Can you work these out from the model? Positions are in its coordinate system, mm. Face numbers are marked on the shaded views. A direction names the side the tool comes from. Coordinates: 2 decimals unless noted, no trailing zeros. Loops run counter-clockwise (first coordinate to the right, second up) from the corner with the lowest first, then second, coordinate; pieces in that order, holes last.
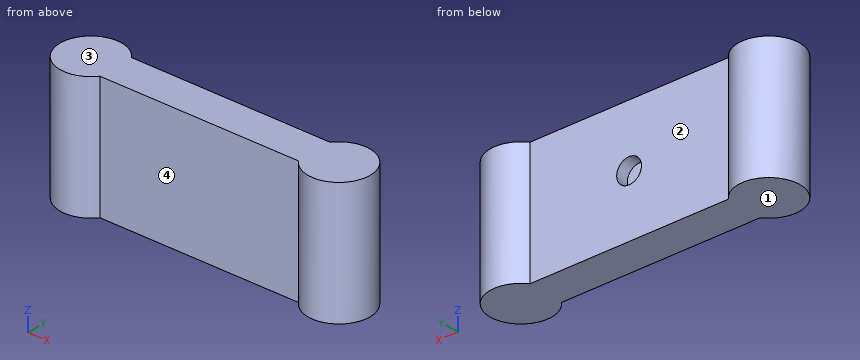
```python
from build123d import *

# Parameters (mm, degrees)
F0_W     = 200
F0_H     = 100
F1_DEPTH = 30
F2_R     = 25
F3_DEPTH = 50
F4_R     = 10
F5_DEPTH = 10


with BuildPart() as f1:
    # F0 (on Front) → F1 (new body)
    with BuildSketch(Plane.XZ):
        Rectangle(F0_W, F0_H)
    extrude(amount=F1_DEPTH)

    # F2 (on Top) → F3 (join, symmetric)
    with BuildSketch(Plane.XY):
        with Locations((-100, -15)):
            Circle(F2_R)
        with Locations((100, -15)):
            Circle(F2_R)
    extrude(amount=F3_DEPTH, both=True)

    # F4 (on Front) → F5 (cut)
    with BuildSketch(Plane.XZ):
        Circle(F4_R)
    extrude(amount=F5_DEPTH, mode=Mode.SUBTRACT)


solid = f1.part
```
Item 1: Suppose I cut it at A-A, the plane x = 0. Please give me the cut outline in (y, z), plus the area to 3 significant figures.
Results are:
outline: (-30, -50) - (0, -50) - (0, -10) - (-10, -10) - (-10, 10) - (0, 10) - (0, 50) - (-30, 50) - close
area: 2,800 mm2
Item 2: I need wall thicknesses on line 1 along Z through (x, y) = (0, -5.5); line 2 along Y through (x, z) = (3.5, 21.5); line 3 along X through (y, z) = (-31, -2). Which ranges of each line are inside material? Lowest first, please.
Results are:
line 1: z = -50 to -10, 10 to 50
line 2: y = -30 to 0
line 3: x = -119.21 to -80.79, 80.79 to 119.21
Item 3: Suppose I cut it at C-C, the plane x = -25. Please give me the cut outline in (y, z), plus the area to 3 significant figures.
Results are:
outline: (-30, -50) - (0, -50) - (0, 50) - (-30, 50) - close
area: 3,000 mm2
Item 4: On a 3-axis mill with a long thin cutter (end or side, diameter ignored), from which of +Z, -Z, +X, -X, +Y, -Y can I reach the whole of each face in a straight line? I mean the marked faces 3 and 4. Say none if no direction works.
Results are:
face 3: +Z, +X, -X, +Y, -Y
face 4: +Z, -Z, -Y
Item 5: Suppose I cut it at D-D, the plane z = -19.5. Please give me the cut outline in (x, y), plus the area to 3 significant figures.
Results are:
outline: (-80, -30) - (80, -30) arc R25 ccw (long way) to (80, 0) - (-80, 0) arc R25 ccw (long way) to start
area: 8,520 mm2
Item 6: We'd pull the mould along X, two halves only. Please class the marked faces 1 and 2: +X half, -X half, draft (parallel to the pull), parting line (faces both ways), or undercut.
Results are:
face 1: draft
face 2: undercut
Item 7: Suppose I cut it at B-B, the plane z = 0. Please give me the cut outline in (x, y), plus the area to 3 significant figures.
Results are:
outline: (-80, -30) - (80, -30) arc R25 ccw (long way) to (80, 0) - (10, 0) - (10, -10) - (-10, -10) - (-10, 0) - (-80, 0) arc R25 ccw (long way) to start
area: 8,320 mm2
Item 8: I'm going to push flat-ended pins straight in: P1, Ø10, axis at y = -1.5, z = -36, coming from the +X side; P2, Ø10, axis at y = -11.5, z = -6, coming from the +X side; P3, Ø12, axis at y = -24.5, z = -18, coming from the -X side. Where does each tip first touch, or does it pass through?
Results are:
P1: stops at x = 123.51
P2: stops at x = 125
P3: stops at x = -124.75
